The listing builds one solid part. Answer for the finished solid, in the listing's coordinates (mm). A direction names the side the tool comes from. Give positions to 0.01 mm unless a question says otherwise; leave off trailing zeros. Order: outer loops, then holes, each group sorted by start corner. A loop starts at its lowest first (then second) coordinate and runs counter-clockwise, first axis right, second up.
```python
from build123d import *

# Parameters (mm, degrees)
SKETCH1_W                       = 101.6
SKETCH1_H                       = 59.436
BASE_EXTRUDE_DEPTH              = 3.81
BASE_CORNER_FILLET_R            = 2.54
SKETCH3_R                       = 1.905
PEG_EXTRUDE_DEPTH               = 2.54
MATERIAL_REMOVAL_CUT_DEPTH      = 120.96788652
SKETCH5_R                       = 1.905
REMOTE_CONTROL_HOLDER_CUT_DEPTH = 120.96788652


with BuildPart() as part:
    # Sketch1 → Base Extrude (new body)
    with BuildSketch(Plane(origin=(0, 0, 0), x_dir=(1, 0, 0), z_dir=(0, 1, 0))):
        with Locations((50.8, 29.718)):
            Rectangle(SKETCH1_W, SKETCH1_H)
    extrude(amount=BASE_EXTRUDE_DEPTH)

    # Base Corner Fillet
    base_corner_fillet_edges = [part.edges().sort_by_distance(p)[0] for p in [
        (0, 1.905, -59.436),
        (101.6, 1.905, -59.436),
        (101.6, 1.905, 0),
        (0, 1.905, 0),
    ]]
    fillet(base_corner_fillet_edges, radius=BASE_CORNER_FILLET_R)

    # Sketch3 → Peg Extrude (add)
    with BuildSketch(Plane.ZY):
        with Locations(Location((-7.493, 1.905, 0), (0, 0, 270))):
            Circle(SKETCH3_R)
        with Locations(Location((-51.943, 1.905, 0), (0, 0, 180))):
            Circle(SKETCH3_R)
    peg_extrude = extrude(amount=PEG_EXTRUDE_DEPTH)

    # Peg Mirror: Peg Extrude across plane
    add(peg_extrude.mirror(Plane(origin=(50.8, 0, 0), x_dir=(0, 0, 1), z_dir=(1, 0, 0))))

    # Sketch4 → Material Removal Cut (cut, through all)
    with BuildSketch(Plane.XZ):
        with BuildLine():
            Line((19.05, -12.7), (82.55, -12.7))
            ThreePointArc((82.55, -12.7), (87.040128061, -14.559871939), (88.9, -19.05))
            Line((88.9, -19.05), (88.9, -40.386))
            ThreePointArc((88.9, -40.386), (87.040128061, -44.876128061), (82.55, -46.736))
            Line((82.55, -46.736), (19.05, -46.736))
            ThreePointArc((19.05, -46.736), (14.559871939, -44.876128061), (12.7, -40.386))
            Line((12.7, -40.386), (12.7, -19.05))
            ThreePointArc((12.7, -19.05), (14.559871939, -14.559871939), (19.05, -12.7))
        make_face()
    extrude(amount=-MATERIAL_REMOVAL_CUT_DEPTH, mode=Mode.SUBTRACT)

    # Sketch5 → Remote Control Holder Cut (cut, through all)
    with BuildSketch(Plane(origin=(0, 3.81, 0), x_dir=(1, 0, 0), z_dir=(0, 1, 0))):
        with Locations(Location((63.5, 4.318, 0), (0, 0, 270))):
            Circle(SKETCH5_R)
        with Locations(Location((63.5, 55.118, 0), (0, 0, 270))):
            Circle(SKETCH5_R)
    extrude(amount=-REMOTE_CONTROL_HOLDER_CUT_DEPTH, mode=Mode.SUBTRACT)


solid = part.part
```
1) Given P1, Ø1.1, axis at y = 2, z = -27, coming from the -X side; P2, Ø1.9, axis at y = 2.5, z = -4, coming from the +X side, each flat-ended and moving along its own axis, determine where each tip first touches the part or whether it passes through.
Geometry says:
P1: stops at x = 0
P2: stops at x = 101.6
2) Find section B-B (z = -27). Write down the section's boundary in (x, y).
Geometry says:
outline: (0, 0) - (12.7, 0) - (12.7, 3.81) - (0, 3.81) - close; (88.9, 0) - (101.6, 0) - (101.6, 3.81) - (88.9, 3.81) - close
3) Find section A-A (x = 81). Write down the section's boundary in (y, z).
Geometry says:
outline: (0, -59.44) - (3.81, -59.44) - (3.81, -46.74) - (0, -46.74) - close; (0, -12.7) - (3.81, -12.7) - (3.81, 0) - (0, 0) - close
4) A tool of negligible diameter and unlimited length cuts with its end or side. For faces 4 (the flat face through (12.7, 2, -30)), 5 (the cylindrical face through (102.85, 3.42, -8.65)), 6 (the cylindrical face through (-1.25, 3.42, -8.65)), from which of +Z, -Z, +X, -X, +Y, -Y can it reach the whole face along a straight path? Write none if from no direction.
Geometry says:
face 4: +Y, -Y
face 5: +X
face 6: -X
5) Find section C-C (x = 63.5). Write down the section's boundary in (y, z).
Geometry says:
outline: (0, -59.44) - (3.81, -59.44) - (3.81, -57.02) - (0, -57.02) - close; (0, -53.21) - (3.81, -53.21) - (3.81, -46.74) - (0, -46.74) - close; (0, -12.7) - (3.81, -12.7) - (3.81, -6.22) - (0, -6.22) - close; (0, -2.41) - (3.81, -2.41) - (3.81, 0) - (0, 0) - close
6) Find section D-D (y = 3.1). Count the separate pieces of the cut face and the enclosed holes in it, then the cut area to 3 significant figures.
Geometry says:
separate pieces: 1
enclosed holes: 3
area: 3,480 mm2
7) Straight lines are drawn through the part: probe 1 along Z at (x, y) = (31.5, 1.55); probe 2 along X at (y, z) = (3, -20); probe 3 along X at (y, z) = (2.2, -55). For each, find the intervals that lie inside material, in ascending order.
Geometry says:
probe 1: z = -59.44 to -46.74, -12.7 to 0
probe 2: x = 0 to 12.7, 88.9 to 101.6
probe 3: x = 0 to 61.6, 65.4 to 101.6
8) For a pull along Z with two mould halves and no side action, classify faces 1 (the cylindrical face through (14.51, 1.88, -14.61)), 2 (the flat face through (104.14, 2, -52)), 3 (the cylindrical face through (0.72, 1.93, -58.67)) as +Z half, -Z half, draft (parallel to the pull), parting line (faces both ways), or undercut.
Geometry says:
face 1: undercut
face 2: draft
face 3: -Z half
